Source: CAD feature listing. Evaluate the final solid. Frame: model axes, mm. A direction names the side the tool comes from. Give positions to 0.01 mm unless a question says otherwise; leave off trailing zeros. Loops run counter-clockwise (first coordinate to the right, second up) from the corner with the lowest first, then second, coordinate; pieces in that order, holes last. Notation, with made-up numbers: M 24,43 L 60,43 A12 cw 60,57 Z; hole C -28,79.25 d1. An arc over 180 degrees is marked long. Put each result on its own line as item: value.
from build123d import *

# Parameters (mm, degrees)
SKETCH1_W           = 31.75
SKETCH1_H           = 31.75
BOSS_EXTRUDE1_DEPTH = 109.855
SHELL1_T            = -3.175
SKETCH2_R           = 4.7625
CUT_EXTRUDE1_DEPTH  = 3.175
SKETCH4_W           = 1.5875
SKETCH4_H           = 3.175
BOSS_EXTRUDE4_DEPTH = 103.505
SKETCH6_W           = 19.05
SKETCH6_H           = 103.505
CUT_EXTRUDE3_DEPTH  = 114.3
SKETCH5_W           = 2.54
SKETCH5_H           = 25.4
CUT_EXTRUDE2_DEPTH  = 106.68
SKETCH8_W           = 19.05
SKETCH8_H           = 3.175
BOSS_EXTRUDE5_DEPTH = 1.5875
SKETCH10_W          = 19.05
SKETCH10_H          = 3.175
BOSS_EXTRUDE7_DEPTH = 1.5875
SKETCH11_W          = 1.5875
SKETCH11_H          = 31.75
BOSS_EXTRUDE8_DEPTH = 103.505
SKETCH13_R          = 6.35
SKETCH13_R_2        = 4.7625
BOSS_EXTRUDE9_DEPTH = 9.525


with BuildPart() as part:
    # Sketch1 → Boss-Extrude1 (new body)
    with BuildSketch(Plane(origin=(0, 0, 0), x_dir=(1, 0, 0), z_dir=(0, 1, 0))):
        Rectangle(SKETCH1_W, SKETCH1_H)
    extrude(amount=BOSS_EXTRUDE1_DEPTH)

    # Shell1
    shell1_openings = [part.faces().sort_by_distance(p)[0] for p in [
        (15.875, 54.9275, 0),
    ]]
    offset(amount=SHELL1_T, openings=shell1_openings, kind=Kind.INTERSECTION)

    # Sketch2 → Cut-Extrude1 (cut)
    with BuildSketch(Plane.XZ):
        Circle(SKETCH2_R)
    extrude(amount=-CUT_EXTRUDE1_DEPTH, mode=Mode.SUBTRACT)

    # Sketch4 → Boss-Extrude4 (add)
    with BuildSketch(Plane(origin=(0, 3.175, 0), x_dir=(1, 0, 0), z_dir=(0, 1, 0))):
        with Locations((15.08125, -11.1125)):
            Rectangle(SKETCH4_W, SKETCH4_H)
        with Locations((15.08125, 11.1125)):
            Rectangle(SKETCH4_W, SKETCH4_H)
        with Locations((10.95375, -11.1125)):
            Rectangle(SKETCH4_W, SKETCH4_H)
        with Locations((10.95375, 11.1125)):
            Rectangle(SKETCH4_W, SKETCH4_H)
        with Locations((-10.95375, 11.1125)):
            Rectangle(SKETCH4_W, SKETCH4_H)
        with Locations((-15.08125, 11.1125)):
            Rectangle(SKETCH4_W, SKETCH4_H)
        with Locations((-15.08125, -11.1125)):
            Rectangle(SKETCH4_W, SKETCH4_H)
        with Locations((-10.95375, -11.1125)):
            Rectangle(SKETCH4_W, SKETCH4_H)
    extrude(amount=BOSS_EXTRUDE4_DEPTH)

    # Sketch6 → Cut-Extrude3 (cut)
    with BuildSketch(Plane(origin=(-12.7, 0, 0), x_dir=(0, 0, -1), z_dir=(1, 0, 0))):
        with Locations((0, 54.9275)):
            Rectangle(SKETCH6_W, SKETCH6_H)
    extrude(amount=-CUT_EXTRUDE3_DEPTH, mode=Mode.SUBTRACT)

    # Sketch5 → Cut-Extrude2 (cut)
    with BuildSketch(Plane(origin=(0, 3.175, 0), x_dir=(1, 0, 0), z_dir=(0, 1, 0))):
        with Locations((13.0175, 0)):
            Rectangle(SKETCH5_W, SKETCH5_H)
        with Locations((-13.0175, 0)):
            Rectangle(SKETCH5_W, SKETCH5_H)
    extrude(amount=CUT_EXTRUDE2_DEPTH, mode=Mode.SUBTRACT)

    # Sketch8 → Boss-Extrude5 (add)
    with BuildSketch(Plane(origin=(15.875, 0, 0), x_dir=(0, 0, -1), z_dir=(1, 0, 0))):
        with Locations((0, 105.0925)):
            Rectangle(SKETCH8_W, SKETCH8_H)
        with Locations((0, 4.7625)):
            Rectangle(SKETCH8_W, SKETCH8_H)
    extrude(amount=-BOSS_EXTRUDE5_DEPTH)

    # Sketch10 → Boss-Extrude7 (add)
    with BuildSketch(Plane.ZY.offset(15.875)):
        with Locations((0, 4.7625)):
            Rectangle(SKETCH10_W, SKETCH10_H)
        with Locations((0, 105.0925)):
            Rectangle(SKETCH10_W, SKETCH10_H)
    extrude(amount=-BOSS_EXTRUDE7_DEPTH)

    # Sketch11 → Boss-Extrude8 (add)
    with BuildSketch(Plane(origin=(0, 109.855, 0), x_dir=(1, 0, 0), z_dir=(0, 1, 0))):
        Rectangle(SKETCH11_W, SKETCH11_H)
    extrude(amount=-BOSS_EXTRUDE8_DEPTH)

    # Sketch13 → Boss-Extrude9 (add)
    with BuildSketch(Plane.XZ):
        Circle(SKETCH13_R)
        Circle(SKETCH13_R_2, mode=Mode.SUBTRACT)
    extrude(amount=BOSS_EXTRUDE9_DEPTH)


solid = part.part
1. Material intervals for line 1 (Z direction, x = 4, y = 40) (3 decimals); line 2 (Z direction, x = 14.5, y = 13) (3 decimals); line 3 (Y direction, x = 11, z = -6.5) (3 decimals), sorted ascending. Write a range as from..to.
Found:
line 1: -15.875..-12.7, 12.7..15.875
line 2: -15.875..-9.525, 9.525..15.875
line 3: 0..3.175, 106.68..109.855
2. Section query C-C (x = 9). Output: boundary loops of the cut face in (y, z) (3 decimals).
Found:
outline: M 0,-15.875 L 109.855,-15.875 L 109.855,15.875 L 0,15.875 Z; hole M 3.175,-12.7 L 106.68,-12.7 L 106.68,12.7 L 3.175,12.7 Z
3. Access query for faces 4 (the flat face through (15.875, 56, 11)), 5 (the flat face through (0, 56, 15.875)), 6 (the flat face through (13, 56, -12.7)), 7 (the cylindrical face through (-3.78, -3.09, -2.9)), 8 (the flat face through (0.794, 57, 0)). Directions: +Z, -Z, +X, -X, +Y, -Y. A direction counts if a zero-diameter tool reaches every point of the face in a straight line with its end or side. Return the directions, or none.
Found:
face 4: +Z, -Z, +X, +Y, -Y
face 5: +Z, +X, -X, +Y, -Y
face 6: +Y
face 7: -Y
face 8: none
4. Section query A-A (z = 0). State how many separate pieces and enclosed holes the cut face has, plus the area to 3 significant figures.
Found:
separate pieces: 5
enclosed holes: 0
area: 365 mm^2
5. Draft query along Y for faces 1 (the flat face through (7, 0, 0)), 2 (the flat face through (-2, 54, 12.7)), 3 (the flat face through (0, 56, -15.875)). Return one class per face: pulls with the +Y half, pulls with the -Y half, needs draft (parallel to the pull), parting line crosses it, or undercut.
Found:
face 1: pulls with the -Y half
face 2: undercut
face 3: needs draft
6. Contact query for flat-ended pins moving along their axis: P1, Ø1.3, axis at x = 15, z = 2.5, coming from the -Y side; P2, Ø4, axis at y = 53, z = -5.5, coming from the -X side; P3, Ø1.5, axis at y = 87.5, z = 6, coming from the +X side. Output: stop coordinate, or through.
Found:
P1: y = 0
P2: x = -0.79
P3: x = 0.79
